Part model, mm, in its own coordinate system. A direction names the side the tool comes from. Coordinates: 2 decimals unless noted, no trailing zeros. Loops run counter-clockwise (first coordinate to the right, second up) from the corner with the lowest first, then second, coordinate; pieces in that order, holes last. Notation, with made-up numbers: M 26,32 L 85,32 A23 ccw 85,51 Z; hole C 1.25,-23 d7. An arc over 180 degrees is marked long. Answer as a JSON object with one key per item and string values. Group by question number.
1. Drop flat-ended pins along their axis: pin 1 Ø12 at (y, z) = (6.5, 96) entering from +X; pin 2 Ø2.5 at (x, z) = (0, 60) entering from -Y; pin 3 Ø8 at (y, z) = (-21.5, 23.5) entering from -X; pin 4 Ø18 at (x, y) = (6.5, -2) entering from +Z. Give the stop position or say it passes through.
2. Drill centre lines: L1, parallel to Z at x = -19, y = -25.5; L2, parallel to Y at x = 0, z = 42.5; L3, parallel to X at y = 5, z = 36.5. Where is each one in solid material? Low to high.
3. Saw through at C-C on z = 68. Write the cut outline in (x, y).
4. Mould opens along Z. For faces 4 (the face through (-0.45, 23.92, 58.57)), 5 (the face through (-6, -21, 0)), 6 (the face through (-29.97, 1.32, 97.18)), 7 (the face through (16, -16, 125)) say: released by +Z, released by -Z, zero draft, split by the parting line, or undercut.
5. Saw through at B-B on x = 0. Count the separate pieces of the cut face and the enclosed holes in it, then the cut area to 3 significant figures.
6. Saw through at D-D on z = 97. Write the cut outline in (x, y), then the cut area to 3 significant figures.
7. 3-axis set-ups, long thin cutter, end or side, ignore diameter. For faces 1 (the face through (-13, -25, 45)), 2 (the face through (-4.336, -19.524, 61.646)), 3 (the face through (-29.97, 1.32, 23.94)): which of +Z, -Z, +X, -X, +Y, -Y reach the whole face in a straight line?
from build123d import *

# Parameters (mm, degrees)
SKETCH1_R               = 30
SKETCH1_R_2             = 20
MAIN_BODY_DEPTH         = 120
SKETCH2_R               = 37.5
SKETCH2_R_2             = 20
BOSS_LIP_DEPTH          = 5
SKETCH4_W               = 4
SKETCH4_H               = 30
BEARLING_CHAMFER_SIZE   = 2
BEARLING_CHAMFER_SIZE2  = 3.464101615
SHAFT_CHAMFER_SIZE      = 1.5
LIP_CHAMFER_SIZE        = 0.75
CUT_EXTRUDE2_REACH      = 137.785
CUT_EXTRUDE2_END_RADIUS = 28
SKETCH5_R               = 1.5


with BuildPart() as part:
    # Sketch1 → Main Body (new body)
    with BuildSketch(Plane.XY):
        Circle(SKETCH1_R)
        Circle(SKETCH1_R_2, mode=Mode.SUBTRACT)
    extrude(amount=MAIN_BODY_DEPTH)

    # Sketch2 → Boss_Lip (add)
    with BuildSketch(Plane.XY.offset(120)):
        Circle(SKETCH2_R)
        Circle(SKETCH2_R_2, mode=Mode.SUBTRACT)
    extrude(amount=BOSS_LIP_DEPTH)

    # Sketch4 → Relief (revolve, cut)
    with BuildSketch(Plane(origin=(0, 0, 0), x_dir=(1, 0, 0), z_dir=(0, 1, 0)), mode=Mode.PRIVATE) as relief_sk:
        with Locations((-30, -60)):
            Rectangle(SKETCH4_W, SKETCH4_H)
    revolve(relief_sk.sketch.rotate(Axis((0, 0, 84), (0, 0, -1)), 180), axis=Axis((0, 0, 84), (0, 0, -1)), mode=Mode.SUBTRACT)

    # Bearling Chamfer
    bearling_chamfer_edges = [part.edges().sort_by_distance(p)[0] for p in [
        (-30, 0, 0),
    ]]
    bearling_chamfer_side = [part.faces().sort_by_distance(p)[0] for p in [
        (-29.151471863, 0, 0),
    ]]
    chamfer(bearling_chamfer_edges, length=BEARLING_CHAMFER_SIZE, length2=BEARLING_CHAMFER_SIZE2, reference=bearling_chamfer_side[0])

    # Shaft Chamfer
    shaft_chamfer_edges = [part.edges().sort_by_distance(p)[0] for p in [
        (-20, 0, 125),
        (-20, 0, 0),
    ]]
    chamfer(shaft_chamfer_edges, length=SHAFT_CHAMFER_SIZE)

    # Lip Chamfer
    lip_chamfer_edges = [part.edges().sort_by_distance(p)[0] for p in [
        (-37.5, 0, 120),
        (-37.5, 0, 125),
    ]]
    chamfer(lip_chamfer_edges, length=LIP_CHAMFER_SIZE)

    # Cut-Extrude2: up to this cylinder (the profile starts inside it)
    cut_extrude2_end = Plane(origin=(0, 0, 60), z_dir=(0, 0, 1)) * Cylinder(CUT_EXTRUDE2_END_RADIUS, 332.57, mode=Mode.PRIVATE)
    # Sketch5 → Cut-Extrude2 (cut, up to the surface)
    with BuildSketch(Plane(origin=(0, 0, 0), x_dir=(1, 0, 0), z_dir=(0, 1, 0)), mode=Mode.PRIVATE) as cut_extrude2_sk1:
        with Locations(Location((0, -60, 0), (0, 0, 90))):
            Circle(SKETCH5_R)
    cut_extrude2_tool1 = extrude(cut_extrude2_sk1.sketch, amount=CUT_EXTRUDE2_REACH, mode=Mode.PRIVATE) & cut_extrude2_end
    add(cut_extrude2_tool1.solids().sort_by_distance((0, 0, 60))[0], mode=Mode.SUBTRACT)


solid = part.part
Outcome:
{
 "1": {"pin 1": "stops at x = 30", "pin 2": "stops at y = -28", "pin 3": "stops at x = -24.37", "pin 4": "passes through"},
 "2": {"L1": "z = 120 to 125", "L2": "y = -30 to -20, 20 to 30", "L3": "x = -29.58 to -19.36, 19.36 to 29.58"},
 "3": {"outline": "C 0,0 d56; hole C 0,0 d40"},
 "4": {"face 4": "undercut", "face 5": "released by -Z", "face 6": "zero draft", "face 7": "released by +Z"},
 "5": {"separate pieces": "3", "enclosed holes": "0", "area": "2,420 mm²"},
 "6": {"outline": "C 0,0 d60; hole C 0,0 d40", "area": "1,570 mm²"},
 "7": {"face 1": "none", "face 2": "+Z, -Z", "face 3": "-Z"}
}
